Could you check a few things on this model? Use its own coordinates, in mm. Face numbers are marked on the shaded views. A direction names the side the tool comes from. Give positions to 0.01 mm unless a question says otherwise; leave off trailing zeros. Write each loop counter-clockwise with the first axis right and the second up, starting at its lowest first coordinate (ties: lowest second). Pieces come first, ordered by that corner, then holes. Notation, with made-up numbers: (-12.5, 12) - (19.5, 12) arc R9 ccw to (19.5, 17) - close; hole circle Ø7 at (47.25, -29). An arc over 180 degrees is marked (long way). Answer as a JSON object with one key per item and string values. Group by question number.
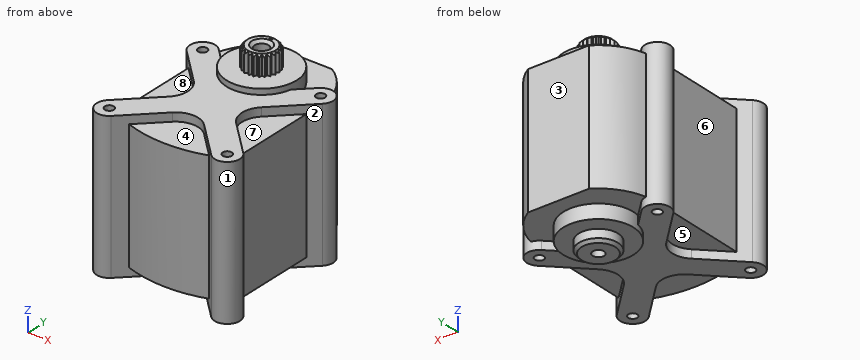
```python
from build123d import *

# Parameters (mm, degrees)
EXTRUDE_1_DEPTH          = 11.5
SKETCH_2_R               = 6.25
EXTRUDE_2_DEPTH          = 14
SKETCH_3_R               = 3.5
EXTRUDE_3_DEPTH          = 2
CHAMFER_1_SIZE           = 0.5
M2_5X0_45_1_D            = 2.05
M2_5X0_45_1_DEPTH        = 7.25
M2_5X0_45_1_TIP          = 0.615882135
EXTRUDE_4_DEPTH          = 13
M2X0_4_1_D               = 1.6
PATTERN_CIRCULAR_1_COUNT = 4
FILLET_1_R               = 4
EXTRUDE_5_DEPTH          = 26
SKETCH_13_R              = 3
EXTRUDE_6_DEPTH          = 3.5
M3X0_5_1_D               = 2.5
M3X0_5_1_DEPTH           = 10
M3X0_5_1_TIP             = 0.751075774
CHAMFER_2_SIZE           = 0.5
SKETCH_17_R              = 0.25
CUT_EXTRUDE_1_DEPTH      = 0.5
CUT_EXTRUDE_2_REACH      = 44.724
PATTERN_CIRCULAR_2_COUNT = 23


with BuildPart() as part:
    # ｽｹｯﾁ1 → ﾎﾞｽ - 押し出し1 (new, symmetric)
    with BuildSketch(Plane.XY):
        with BuildLine():
            Line((-5.408326913, 9), (5.408326913, 9))
            ThreePointArc((5.408326913, 9), (9.138857494, 5.170230527), (10.5, 0))
            Line((10.5, 0), (10.5, -19.332614929))
            ThreePointArc((10.5, -19.332614929), (0, -22), (-10.5, -19.332614929))
            Line((-10.5, -19.332614929), (-10.5, 0))
            ThreePointArc((-10.5, 0), (-9.138857494, 5.170230527), (-5.408326913, 9))
        make_face()
    extrude(amount=EXTRUDE_1_DEPTH, both=True)

    # ｽｹｯﾁ2 → ﾎﾞｽ - 押し出し2 (add, symmetric)
    with BuildSketch(Plane.XY):
        Circle(SKETCH_2_R)
    extrude(amount=EXTRUDE_2_DEPTH, both=True)

    # ｽｹｯﾁ3 → ﾎﾞｽ - 押し出し3 (add)
    with BuildSketch(Plane(origin=(0, 0, -14), x_dir=(-1, 0, 0), z_dir=(0, 0, -1))):
        Circle(SKETCH_3_R)
    extrude(amount=EXTRUDE_3_DEPTH)

    # 面取り1
    chamfer_1_edges = [part.edges().sort_by_distance(p)[0] for p in [
        (3.5, 0, -16),
    ]]
    chamfer(chamfer_1_edges, length=CHAMFER_1_SIZE)

    # M2.5x0.45 ねじ穴1
    with Locations(Plane(origin=(0, 0, -16), x_dir=(-1, 0, 0), z_dir=(0, 0, -1))):
        with Locations((0, 0)):
            Hole(M2_5X0_45_1_D / 2, depth=M2_5X0_45_1_DEPTH)
            with Locations((0, 0, -(M2_5X0_45_1_DEPTH + M2_5X0_45_1_TIP / 2))):  # 118° drill point
                Cone(0, M2_5X0_45_1_D / 2, M2_5X0_45_1_TIP, mode=Mode.SUBTRACT)

    # ｽｹｯﾁ7 → ﾎﾞｽ - 押し出し4 (add, symmetric)
    with BuildSketch(Plane.XY):
        with BuildLine():
            Line((-12.090990258, -1.590990258), (-3.181980515, -10.5))
            Line((-3.181980515, -10.5), (0, -10.5))
            Line((0, -10.5), (0, -7.318019485))
            Line((0, -7.318019485), (-8.909009742, 1.590990258))
            ThreePointArc((-8.909009742, 1.590990258), (-12.090990258, 1.590990258), (-12.090990258, -1.590990258))
        make_face()
    extrude_4 = extrude(amount=EXTRUDE_4_DEPTH, both=True)

    # M2x0.4 ねじ穴1 (through all)
    with Locations(Plane.XY.offset(13)):
        with Locations((-10.5, 0)):
            m2x0_4_1 = Hole(M2X0_4_1_D / 2)

    # 円形ﾊﾟﾀｰﾝ1: ﾎﾞｽ - 押し出し4, M2x0.4 ねじ穴1 ×4 about axis
    pattern_circular_1_axis = Axis((0, -10.5, 0), (0, 0, 1))
    add([extrude_4.rotate(pattern_circular_1_axis, i * 360 / PATTERN_CIRCULAR_1_COUNT) for i in range(1, PATTERN_CIRCULAR_1_COUNT)])
    add([m2x0_4_1.rotate(pattern_circular_1_axis, i * 360 / PATTERN_CIRCULAR_1_COUNT) for i in range(1, PATTERN_CIRCULAR_1_COUNT)], mode=Mode.SUBTRACT)

    # ﾌｨﾚｯﾄ1
    fillet_1_edges = [part.edges().sort_by_distance(p)[0] for p in [
        (3.181980515, -10.5, -12.25),
        (3.181980515, -10.5, 12.25),
        (0, -13.681980515, -12.25),
        (0, -13.681980515, 12.25),
        (-3.181980515, -10.5, -12.25),
        (-3.181980515, -10.5, 12.25),
    ]]
    fillet(fillet_1_edges, radius=FILLET_1_R)

    # ｽｹｯﾁ12 → ﾎﾞｽ - 押し出し5 (add)
    with BuildSketch(Plane(origin=(0, 0, -13), x_dir=(-1, 0, 0), z_dir=(0, 0, -1))):
        Polygon((0, -7.318019485), (-1.180522763, -6.137496721), (1.180522763, -6.137496721), align=None)
    extrude(amount=-EXTRUDE_5_DEPTH)

    # ｽｹｯﾁ13 → ﾎﾞｽ - 押し出し6 (add)
    with BuildSketch(Plane.XY.offset(14)):
        Circle(SKETCH_13_R)
    extrude(amount=EXTRUDE_6_DEPTH)

    # M3x0.5 ねじ穴1
    with Locations(Plane.XY.offset(17.5)):
        with Locations((0, 0)):
            Hole(M3X0_5_1_D / 2, depth=M3X0_5_1_DEPTH)
            with Locations((0, 0, -(M3X0_5_1_DEPTH + M3X0_5_1_TIP / 2))):  # 118° drill point
                Cone(0, M3X0_5_1_D / 2, M3X0_5_1_TIP, mode=Mode.SUBTRACT)

    # 面取り2
    chamfer_2_edges = [part.edges().sort_by_distance(p)[0] for p in [
        (-3, 0, 17.5),
        (1.25, 0, 17.5),
    ]]
    chamfer(chamfer_2_edges, length=CHAMFER_2_SIZE)

    # ｽｹｯﾁ17 → ｶｯﾄ - 押し出し1 (cut)
    with BuildSketch(Plane.XY.offset(17.5)):
        with Locations((0, 2)):
            Circle(SKETCH_17_R)
    extrude(amount=-CUT_EXTRUDE_1_DEPTH, mode=Mode.SUBTRACT)

    # ｶｯﾄ - 押し出し2: up to this face of the body (flat: up to its plane)
    cut_extrude_2_end = Plane(part.part.faces().sort_by_distance((-6.073223305, 0, 14))[0])
    # ｽｹｯﾁ18 → ｶｯﾄ - 押し出し2 (cut, up to the picked face)
    with BuildSketch(Plane.XY.offset(17.5), mode=Mode.PRIVATE) as cut_extrude_2_sk1:
        with BuildLine():
            Line((0, 2.574530741), (-0.408499947, 2.972057838))
            Line((-0.408499947, 2.972057838), (-0.476583272, 3.467400811))
            ThreePointArc((-0.476583272, 3.467400811), (0, 3.5), (0.476583272, 3.467400811))
            Line((0.476583272, 3.467400811), (0.408499947, 2.972057838))
            Line((0.408499947, 2.972057838), (0, 2.574530741))
        make_face()
    cut_extrude_2_tool1 = split(extrude(cut_extrude_2_sk1.sketch, amount=-CUT_EXTRUDE_2_REACH, mode=Mode.PRIVATE), bisect_by=cut_extrude_2_end, keep=Keep.BOTH, mode=Mode.PRIVATE)
    cut_extrude_2 = cut_extrude_2_tool1.solids().sort_by(Axis((0, 3.133577, 17.5), (0, 0, -1)))[0]
    add(cut_extrude_2, mode=Mode.SUBTRACT)

    # 円形ﾊﾟﾀｰﾝ2: ｶｯﾄ - 押し出し2 ×23 about axis
    pattern_circular_2_axis = Axis((0, 0, 0), (0, 0, 1))
    for i in range(1, PATTERN_CIRCULAR_2_COUNT):
        add(cut_extrude_2.rotate(pattern_circular_2_axis, i * 360 / PATTERN_CIRCULAR_2_COUNT), mode=Mode.SUBTRACT)


solid = part.part
```
(1) I need wall thicknesses on L1, parallel to Y at x = 0, z = 10; L2, parallel to Z at x = 9, y = -10; L3, parallel to Z at x = -0.25, y = -15. Which ranges of each line are inside material? Lowest first, please.
(2) Will these pins go through, and if not, where does the flat tip stop? P1, Ø1.5, axis at x = 5, y = -2.5, coming from the +Z side; P2, Ø3, axis at x = 0, y = 0, coming from the +Z side; P3, Ø1.5, axis at x = 9.5, y = -18, coming from the +Z side.
(3) I want a section at C-C, the plane z = 4. Please give me the cut outline in (x, y), and give its area (3 significant figures).
(4) I want a section at B-B, the plane y = -10.5. Please give me the cut outline in (x, z).
(5) If we mould it in two halves opening along X, with no side actions, what happens to the marked faces 1, 2 and 3? For each: +X half, -X half, draft (parallel to the pull), parting line (faces both ways), or undercut.
(6) For the marked faces 4, 5, 6, 7 and 8, which set-ups out of +Z, -Z, +X, -X, +Y, -Y let a thin tool reach every point of the face, with its end or its side?
(7) I want a section at D-D, the plane x = 8.25. Please give me the cut outline in (y, z), and give its area (3 significant figures).
(8) I want a section at A-A, the plane z = -10. Please give me the cut outline in (x, y) (3 decimals), and give its area (3 significant figures).
Entries:
{
 "1": {"L1": "-22 to -1.25, 1.25 to 9", "L2": "-11.5 to 11.5", "L3": "-13 to 13"},
 "2": {"P1": "z = 14", "P2": "z = 17.25", "P3": "z = 13"},
 "3": {"outline": "(-12.09, -19.41) arc R2.25 ccw to (-8.91, -22.59) - (-7.13, -20.81) arc R22 ccw to (7.13, -20.81) - (8.91, -22.59) arc R2.25 ccw to (12.09, -19.41) - (10.5, -17.82) - (10.5, -3.18) - (12.09, -1.59) arc R2.25 ccw to (10.26, 2.24) arc R10.5 ccw to (5.41, 9) - (-5.41, 9) arc R10.5 ccw to (-10.26, 2.24) arc R2.25 ccw to (-12.09, -1.59) - (-10.5, -3.18) - (-10.5, -17.82) - close; hole circle Ø1.6 at (-10.5, -21); hole circle Ø1.6 at (-10.5, 0); hole circle Ø1.6 at (10.5, -21); hole circle Ø1.6 at (10.5, 0)", "area": "647 mm^2"},
 "4": {"outline": "(-10.5, -11.5) - (-4.84, -11.5) - (-4.84, -13) - (4.84, -13) - (4.84, -11.5) - (10.5, -11.5) - (10.5, 11.5) - (4.84, 11.5) - (4.84, 13) - (-4.84, 13) - (-4.84, 11.5) - (-10.5, 11.5) - close"},
 "5": {"face 1": "undercut", "face 2": "+X half", "face 3": "draft"},
 "6": {"face 4": "+Z, -Y", "face 5": "-Z, -X", "face 6": "+Z, -Z, -X", "face 7": "+Z, +X", "face 8": "+Z, -X"},
 "7": {"outline": "(-21.93, -13) - (-15.57, -13) - (-15.57, -11.5) - (-5.43, -11.5) - (-5.43, -13) - (0.93, -13) - (0.93, -11.5) - (6.5, -11.5) - (6.5, 11.5) - (0.93, 11.5) - (0.93, 13) - (-5.43, 13) - (-5.43, 11.5) - (-15.57, 11.5) - (-15.57, 13) - (-21.93, 13) - close", "area": "692 mm^2"},
 "8": {"outline": "(-12.091, -19.409) arc R2.25 ccw to (-8.909, -22.591) - (-7.13, -20.812) arc R22 ccw to (7.13, -20.812) - (8.909, -22.591) arc R2.25 ccw to (12.091, -19.409) - (10.5, -17.818) - (10.5, -3.182) - (12.091, -1.591) arc R2.25 ccw to (10.259, 2.237) arc R10.5 ccw to (5.408, 9) - (-5.408, 9) arc R10.5 ccw to (-10.259, 2.237) arc R2.25 ccw to (-12.091, -1.591) - (-10.5, -3.182) - (-10.5, -17.818) - close; hole circle Ø1.6 at (-10.5, -21); hole circle Ø1.6 at (-10.5, 0); hole circle Ø2.05 at (0, 0); hole circle Ø1.6 at (10.5, -21); hole circle Ø1.6 at (10.5, 0)", "area": "644 mm^2"}
}
